from build123d import *

# Parameters (mm, degrees)
SKETCH2_R           = 8.5
SKETCH2_R_2         = 1
SKETCH2_R_3         = 1.55
SKETCH2_W           = 2.6
SKETCH2_H           = 52
SKETCH2_W_2         = 15
SKETCH2_H_2         = 15
BOSS_EXTRUDE1_DEPTH = 2.5


with BuildPart() as part:
    # Sketch2 → Boss-Extrude1 (new body)
    with BuildSketch(Plane(origin=(0, 0, 0), x_dir=(1, 0, 0), z_dir=(0, 1, 0))):
        Polygon((-25, 35), (-77.6, 35), (-77.6, -35), (-25, -35), (-25, -39), (25, -39), (25, -35), (77.6, -35), (77.6, 35), (25, 35), (25, 39), (-25, 39), align=None)
        with Locations((-12.5, 12.818198975)):
            Circle(SKETCH2_R, mode=Mode.SUBTRACT)
        with Locations((-21, 21.318198975)):
            Circle(SKETCH2_R_2, mode=Mode.SUBTRACT)
        with Locations((-21, 4.318198975)):
            Circle(SKETCH2_R_2, mode=Mode.SUBTRACT)
        with Locations((21, 4.318198975)):
            Circle(SKETCH2_R_2, mode=Mode.SUBTRACT)
        with Locations((21, 21.318198975)):
            Circle(SKETCH2_R_2, mode=Mode.SUBTRACT)
        with Locations((12.5, 12.818198975)):
            Circle(SKETCH2_R, mode=Mode.SUBTRACT)
        with Locations((-42.5, -7.181801025)):
            Circle(SKETCH2_R_3, mode=Mode.SUBTRACT)
        with Locations((42.5, -7.181801025)):
            Circle(SKETCH2_R_3, mode=Mode.SUBTRACT)
        with Locations((-73.3, 0)):
            Rectangle(SKETCH2_W, SKETCH2_H, mode=Mode.SUBTRACT)
        with Locations((73.3, 0)):
            Rectangle(SKETCH2_W, SKETCH2_H, mode=Mode.SUBTRACT)
        with Locations((42.5, 12.818198975)):
            Rectangle(SKETCH2_W_2, SKETCH2_H_2, mode=Mode.SUBTRACT)
        with Locations((-42.5, 12.818198975)):
            Rectangle(SKETCH2_W_2, SKETCH2_H_2, mode=Mode.SUBTRACT)
    extrude(amount=BOSS_EXTRUDE1_DEPTH)


solid = part.part
Work out the finished part from the listing and answer in its coordinate system (mm). Give positions to 0.01 mm unless a question says otherwise; leave off trailing zeros. Order: outer loops, then holes, each group sorted by start corner. A loop starts at its lowest first (then second) coordinate and runs counter-clockwise, first axis right, second up. Notation, with made-up numbers: (-15.5, 42) -> (36.5, 42) arc R23 ccw to (36.5, 70) -> close; hole circle Ø6 at (50, -2.75). An arc over 180 degrees is marked (long way). One line per item, written item: value.
Item 1: Determine the mould class of faces 1 (the cylindrical face through (-18.765, 1.232, -18.563)), 2 (the flat face through (-1, 0, -1)) for opening direction X: released by +X, released by -X, zero draft, split by the parting line, or undercut.
Answer sheet:
face 1: undercut
face 2: zero draft
Item 2: Find section D-D, the plane x = -12.5. Give the vertices of the cut face in (y, z).
Answer sheet:
outline: (0, -39) -> (2.5, -39) -> (2.5, -21.32) -> (0, -21.32) -> close; (0, -4.32) -> (2.5, -4.32) -> (2.5, 39) -> (0, 39) -> close
Item 3: Find section B-B, the plane x = 38. Give the vertices of the cut face in (y, z).
Answer sheet:
outline: (0, -35) -> (2.5, -35) -> (2.5, -20.32) -> (0, -20.32) -> close; (0, -5.32) -> (2.5, -5.32) -> (2.5, 35) -> (0, 35) -> close
Item 4: Find section A-A, the plane x = -42.5. Give the vertices of the cut face in (y, z).
Answer sheet:
outline: (0, -35) -> (2.5, -35) -> (2.5, -20.32) -> (0, -20.32) -> close; (0, -5.32) -> (2.5, -5.32) -> (2.5, 5.63) -> (0, 5.63) -> close; (0, 8.73) -> (2.5, 8.73) -> (2.5, 35) -> (0, 35) -> close
Item 5: Straight lines are drawn through the part: probe 1 along X at (y, z) = (0.15, 23.5); probe 2 along Z at (x, y) = (-42.5, 1.25); probe 3 along Z at (x, y) = (-12.5, 1). For each, find the intervals that lie inside material, in ascending order.
Answer sheet:
probe 1: -77.6 to -74.6, -72 to 72, 74.6 to 77.6
probe 2: -35 to -20.32, -5.32 to 5.63, 8.73 to 35
probe 3: -39 to -21.32, -4.32 to 39
Item 6: Find section C-C, the plane z = -17. Give the vertices of the cut face in (x, y), plus the area to 3 significant figures.
Answer sheet:
outline: (-77.6, 0) -> (-74.6, 0) -> (-74.6, 2.5) -> (-77.6, 2.5) -> close; (-72, 0) -> (-50, 0) -> (-50, 2.5) -> (-72, 2.5) -> close; (-35, 0) -> (-19.9, 0) -> (-19.9, 2.5) -> (-35, 2.5) -> close; (-5.1, 0) -> (5.1, 0) -> (5.1, 2.5) -> (-5.1, 2.5) -> close; (19.9, 0) -> (35, 0) -> (35, 2.5) -> (19.9, 2.5) -> close; (50, 0) -> (72, 0) -> (72, 2.5) -> (50, 2.5) -> close; (74.6, 0) -> (77.6, 0) -> (77.6, 2.5) -> (74.6, 2.5) -> close
area: 226 mm²
Item 7: Flat-ended cylindrical pins translate along their axes: P1, Ø2.5, axis at x = 21, z = -4.32, coming from the -Y side; P2, Ø1.2, axis at x = 60.5, y = 1.5, coming from the -Z side; P3, Ø1.2, axis at y = 0.5, z = 36.5, coming from the +X side; P4, Ø1.2, axis at y = 1, z = 37.5, coming from the -X side. Find the tip coordinate at first contact, or state that the pin passes through.
Answer sheet:
P1: y = 0
P2: z = -35
P3: x = 25
P4: x = -25
